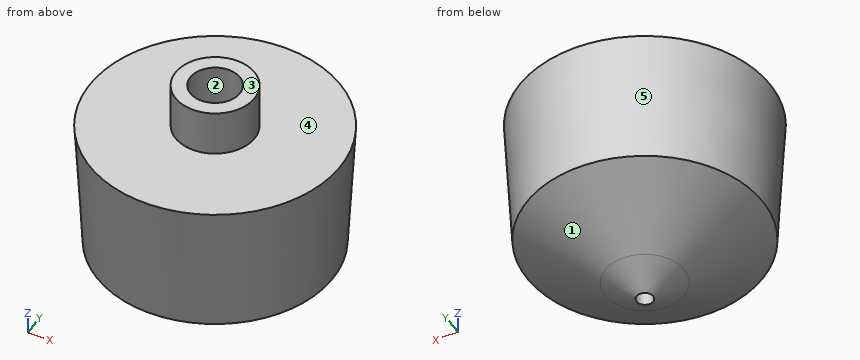
from build123d import *

# Parameters (mm, degrees)
F2_R     = 4.7752
F3_DEPTH = 12.7
F4_R     = 1.6002
F5_DEPTH = 19.685


with BuildPart() as f1:
    # F0 (on Front) → F1 (revolve)
    with BuildSketch(Plane.XZ):
        Polygon((0, 48.26), (0, 0), (7.62, 4.57905), (22.692223, 14.010726), (24.13, 39.37), (7.62, 39.37), (7.62, 48.26), align=None)
    revolve(axis=Axis((0, 0, 24.13), (0, 0, -1)))

    # F2 (on face) → F3 (cut)
    with BuildSketch(Plane.XY.offset(48.26)):
        Circle(F2_R)
    extrude(amount=-F3_DEPTH, mode=Mode.SUBTRACT)

    # F4 (on Top) → F5 (cut)
    with BuildSketch(Plane.XY):
        Circle(F4_R)
    extrude(amount=F5_DEPTH, mode=Mode.SUBTRACT)


solid = f1.part
The listing builds one solid part. Answer for the finished solid, in the listing's coordinates (mm). Face numbers are marked on the shaded views. A direction names the side the tool comes from. Give positions to 0.01 mm unless a question says otherwise; leave off trailing zeros. Order: outer loops, then holes, each group sorted by start corner. A loop starts at its lowest first (then second) coordinate and runs counter-clockwise, first axis right, second up. Notation, with made-up numbers: (28, 88.25) - (40, 88.25) arc R22 cw to (40, 99.25) - close; hole circle Ø11 at (87.25, 6.25). An arc over 180 degrees is marked (long way). Answer as CSV lines item,"result".
Q1. A cutting plane is placed at C-C, the plane z = 16.5. Determine the outline of the cut face in (x, y).
Answer key:
outline,"circle Ø45.67 at (0, 0); hole circle Ø3.2 at (0, 0)"
Q2. A cutting plane is placed at D-D, the plane z = 30. Determine the outline of the cut face in (x, y), and give its area (3 significant figures).
Answer key:
outline,"circle Ø47.2 at (0, 0)"
area,"1,750 mm^2"
Q3. Each of these flat-tipped pins is pushed along its axis until it touches: pin 1 Ø12 at (x, y) = (-5.5, -5.5) entering from -Z; pin 2 Ø8 at (y, z) = (11, 25) entering from +X; pin 3 Ø1 at (y, z) = (-2, 42) entering from -X. Where does it stop, or does it pass through?
Answer key:
pin 1,"stops at z = 1.07"
pin 2,"stops at x = 22.26"
pin 3,"stops at x = -7.47"
Q4. Straight lines are drawn through the part: L1, parallel to Y at x = 0, z = 43; L2, parallel to Y at x = 0, z = 8; L3, parallel to X at y = -1, z = 45.5. For each, find the intervals that lie inside material, in ascending order.
Answer key:
L1,"y = -7.62 to -4.78, 4.78 to 7.62"
L2,"y = -13.09 to -1.6, 1.6 to 13.09"
L3,"x = -7.55 to -4.67, 4.67 to 7.55"
Q5. A cutting plane is placed at A-A, the plane y = 0. Determine the outline of the cut face in (x, z) (3 decimals), and give its area (3 significant figures).
Answer key:
outline,"(-24.13, 39.37) - (-22.692, 14.011) - (-7.62, 4.579) - (-1.6, 0.962) - (-1.6, 19.685) - (1.6, 19.685) - (1.6, 0.962) - (7.62, 4.579) - (22.692, 14.011) - (24.13, 39.37) - (7.62, 39.37) - (7.62, 48.26) - (4.775, 48.26) - (4.775, 35.56) - (-4.775, 35.56) - (-4.775, 48.26) - (-7.62, 48.26) - (-7.62, 39.37) - close"
area,"1,460 mm^2"
Q6. Which of the six approach directions +Z, -Z, +X, -X, +Y, -Y give full straight-line access (tool end or side, diameter ignored) to the marked faces 4 and 5?
Answer key:
face 4,"+Z"
face 5,"-Z"
Q7. Determine the mould class of the marked faces 1, 2 and 3 for opening direction X: pulls with the +X half, pulls with the -X half, needs draft (parallel to the pull), parting line crosses it, or undercut.
Answer key:
face 1,"parting line crosses it"
face 2,"undercut"
face 3,"needs draft"
